from build123d import *

# Parameters (mm, degrees)
F0_W     = 25.4
F0_H     = 38.1
F1_DEPTH = 38.1
F2_T     = -6.325
F3_DEPTH = 19.075
F4_DEPTH = 114.3
F6_D     = 6.5
F6_DEPTH = 50
F6_TIP   = 1.9527970118
F7_W     = 6.325
F7_H     = 76.2
F8_W     = 6.325
F8_H     = 76.2
F9_DEPTH = 31.775


with BuildPart() as f1:
    # F0 (on Top) → F1 (new body)
    with BuildSketch(Plane.XY):
        Rectangle(F0_W, F0_H)
    extrude(amount=F1_DEPTH)

    # F2
    f2_openings = [f1.faces().sort_by_distance(p)[0] for p in [
        (0, 19.05, 19.05),
        (0, 0, 38.1),
        (0, 0, 0),
    ]]
    offset(amount=F2_T, openings=f2_openings)

    # F3 (add): a face of the model
    f3_faces = [f1.faces().sort_by_distance(p)[0] for p in [
        (0, -19.05, 19.05),
    ]]
    extrude(f3_faces, amount=F3_DEPTH)

    # F4 (add): a face of the model
    f4_faces = [f1.faces().sort_by_distance(p)[0] for p in [
        (0, -14.4511656595, 0),
    ]]
    extrude(f4_faces, amount=F4_DEPTH)

    # F6
    with Locations(Plane(origin=(0, -12.725, 0), x_dir=(-1, 0, 0), z_dir=(0, 1, 0))):
        with Locations((0, -104.775), (0, 28.575)):
            Hole(F6_D / 2, depth=F6_DEPTH)
            with Locations((0, 0, -(F6_DEPTH + F6_TIP / 2))):  # 118° drill point
                Cone(0, F6_D / 2, F6_TIP, mode=Mode.SUBTRACT)

    # F7 (on face) + F8 (on face) → F9 (cut)
    with BuildSketch(Plane(origin=(0, 19.05, 0), x_dir=(-1, 0, 0), z_dir=(0, 1, 0))):
        with Locations((-9.5375, -38.1)):
            Rectangle(F7_W, F7_H)
    with BuildSketch(Plane(origin=(0, 19.05, 0), x_dir=(-1, 0, 0), z_dir=(0, 1, 0))):
        with Locations((9.5375, -38.1)):
            Rectangle(F8_W, F8_H)
    extrude(amount=-F9_DEPTH, mode=Mode.SUBTRACT)


solid = f1.part
Model file for the job. Use its own axes, mm. A direction names the side the tool comes from. Give positions to 0.01 mm unless a question says otherwise; leave off trailing zeros. Order: outer loops, then holes, each group sorted by start corner. A loop starts at its lowest first (then second) coordinate and runs counter-clockwise, first axis right, second up. Notation, with made-up numbers: (75, -35) - (117, -35) arc R38 ccw to (117, 4) - close; hole circle Ø4 at (40, 4.25). An arc over 180 degrees is marked (long way). Write item = value, one per line. Start each with the question number.
1. Cut at A-A, the plane y = 7. List the corners of the cut face in (x, z) (3 decimals), and give its area (3 significant figures).
2. Cut at B-B, the plane x = 0. List the corners of the cut face in (y, z) (3 decimals), and give its area (3 significant figures).
3. Cut at D-D, the plane z = -9. List the corners of the cut face in (x, y) (3 decimals), and give its area (3 significant figures).
4. Drop flat-ended pins along their axis: P1, Ø10, axis at x = -4, z = -48, coming from the +Y side (3 decimals); P2, Ø6, axis at x = 4.5, y = -12, coming from the -Z side. Give the stop position or say it passes through.
5. Which spindle directions (+Z, -Z, +X, -X, +Y, -Y) get a long thin tool onto all of the face, cutting with end or side? Do faces 1 (the flat face through (0, -15, -114.3)), 2 (the flat face through (-9, 3, 0)), 3 (the flat face through (-6.375, 3, 19)). Say none if no direction does.
6. Two-plate mould, pull along X, no slides. Class faces 4 (the cylindrical face through (-0.423, -25.603, -101.553)), 5 (the flat face through (10, 3, 0)), 6 (the flat face through (12.7, -15, -37)): pulls with the +X half, pulls with the -X half, needs draft (parallel to the pull), parting line crosses it, or undercut.
7. Cut at C-C, the plane x = 8.75. List the corners of the cut face in (y, z) (3 decimals), and give its area (3 significant figures).
8. Probe line 1 along Z through (x, y) = (0, -21.5) (3 decimals); line 2 along X through (y, z) = (-5, -106) (3 decimals); line 3 along Z through (x, y) = (10.75, 9). List the from-to ranges inside material, lowest first.
Taken from the geometry:
q1.outline = (-12.7, -114.3) - (-6.375, -114.3) - (-6.375, -76.2) - (-12.7, -76.2) - close; (-12.7, 0) - (-6.375, 0) - (-6.375, 38.1) - (-12.7, 38.1) - close; (6.375, -114.3) - (12.7, -114.3) - (12.7, -76.2) - (6.375, -76.2) - close; (6.375, 0) - (12.7, 0) - (12.7, 38.1) - (6.375, 38.1) - close
q1.area = 964 mm²
q2.outline = (-38.125, -114.3) - (-12.725, -114.3) - (-12.725, -108.025) - (-38.125, -108.025) - close; (-38.125, -101.525) - (-12.725, -101.525) - (-12.725, 25.325) - (-38.125, 25.325) - close; (-38.125, 31.825) - (-12.725, 31.825) - (-12.725, 38.1) - (-38.125, 38.1) - close
q2.area = 3,540 mm²
q3.outline = (-12.7, -38.125) - (12.7, -38.125) - (12.7, -12.725) - (-12.7, -12.725) - close
q3.area = 645 mm²
q4.P1 = -12.725
q4.P2 = -114.3
q5.face_1 = -Z, +X, -X, +Y, -Y
q5.face_2 = +X, -X, +Y
q5.face_3 = +Z, -Z, +Y
q6.face_4 = undercut
q6.face_5 = needs draft
q6.face_6 = pulls with the +X half
q7.outline = (-38.125, -114.3) - (19.05, -114.3) - (19.05, -76.2) - (-12.725, -76.2) - (-12.725, 0) - (19.05, 0) - (19.05, 38.1) - (-38.125, 38.1) - close
q7.area = 6,290 mm²
q8.line_1 = -114.3 to -108.025, -101.525 to 25.325, 31.825 to 38.1
q8.line_2 = -12.7 to -6.375, 6.375 to 12.7
q8.line_3 = -114.3 to -76.2, 0 to 38.1
